Model file for the job. Use its own axes, mm. A direction names the side the tool comes from. Round coordinates to 2 decimals unless told otherwise and drop trailing zeros. Write each loop counter-clockwise with the first axis right and the second up, starting at its lowest first coordinate (ties: lowest second). Pieces come first, ordered by that corner, then holes.
```python
from build123d import *

# Parameters (mm, degrees)
SKETCH1_W                       = 210
SKETCH1_H                       = 120
CHASIS_BASE_DEPTH               = 3
FRONT_AND_BACK_SLOTS_DEPTH      = 279.202975413
FRONT_AND_BACK_SLOTS_DEPTH_BACK = 279.202975413
SKETCH7_W                       = 50
SKETCH7_H                       = 3
BACK_WHEELS_DEPTH               = 279.202975413
BACK_WHEELS_DEPTH_BACK          = 279.202975413
CUT_EXTRUDE1_DEPTH              = 279.202975413
CUT_EXTRUDE1_DEPTH_BACK         = 279.202975413
SKETCH16_W                      = 3
SKETCH16_H                      = 10.9
SKETCH17_W                      = 210
SKETCH17_H                      = 30.004914443
CUT_EXTRUDE2_DEPTH              = 10
SKETCH18_W                      = 80
SKETCH18_H                      = 65
CUT_EXTRUDE3_DEPTH              = 57
CUT_EXTRUDE4_DEPTH              = 10
BOSS_EXTRUDE1_DEPTH             = 3


with BuildPart() as part:
    # Sketch1 → Chasis Base (new body)
    with BuildSketch(Plane(origin=(0, 0, 0), x_dir=(1, 0, 0), z_dir=(0, 1, 0))):
        with Locations((-50.389260457, -170.742439233)):
            Rectangle(SKETCH1_W, SKETCH1_H)
    extrude(amount=CHASIS_BASE_DEPTH)

    # Sketch7 → Front and Back Slots (cut, two sides: drawn at the far end of the back side and taken through both)
    with BuildSketch(Plane(origin=(0, 3, 0), x_dir=(1, 0, 0), z_dir=(0, 1, 0)).offset(-FRONT_AND_BACK_SLOTS_DEPTH_BACK)):
        with Locations((-0.389260457, -229.242439233)):
            Rectangle(SKETCH7_W, SKETCH7_H)
        with Locations((-100.389260457, -229.242439233)):
            Rectangle(SKETCH7_W, SKETCH7_H)
    extrude(amount=FRONT_AND_BACK_SLOTS_DEPTH + FRONT_AND_BACK_SLOTS_DEPTH_BACK, mode=Mode.SUBTRACT)

    # Sketch15 → Back Wheels (cut, two sides: drawn at the far end of the back side and taken through both)
    with BuildSketch(Plane(origin=(0, 3, 0), x_dir=(1, 0, 0), z_dir=(0, 1, 0)).offset(-BACK_WHEELS_DEPTH_BACK)):
        Polygon((-155.389260457, -175.747353676), (-155.389260457, -140.747353676), (-127.889260457, -140.747353676), (-127.889260457, -210.747353676), (-155.389260457, -210.747353676), align=None)
        Polygon((54.610739543, -140.747353676), (27.110739543, -140.747353676), (27.110739543, -210.747353676), (54.610739543, -210.747353676), (54.610739543, -175.747353676), align=None)
    extrude(amount=BACK_WHEELS_DEPTH + BACK_WHEELS_DEPTH_BACK, mode=Mode.SUBTRACT)

    # Sketch16 → Cut-Extrude1 (cut, two sides: drawn at the far end of the back side and taken through both)
    with BuildSketch(Plane(origin=(0, 3, 0), x_dir=(1, 0, 0), z_dir=(0, 1, 0)).offset(-CUT_EXTRUDE1_DEPTH_BACK)):
        with Locations((-104.589260457, -155.177353676)):
            Rectangle(SKETCH16_W, SKETCH16_H)
        with Locations((3.810739543, -155.177353676)):
            Rectangle(SKETCH16_W, SKETCH16_H)
    extrude(amount=CUT_EXTRUDE1_DEPTH + CUT_EXTRUDE1_DEPTH_BACK, mode=Mode.SUBTRACT)

    # Sketch17 → Cut-Extrude2 (cut)
    with BuildSketch(Plane(origin=(0, 3, 0), x_dir=(1, 0, 0), z_dir=(0, 1, 0))):
        with Locations((-50.389260457, -125.744896455)):
            Rectangle(SKETCH17_W, SKETCH17_H)
    extrude(amount=-CUT_EXTRUDE2_DEPTH, mode=Mode.SUBTRACT)

    # Sketch18 → Cut-Extrude3 (cut)
    with BuildSketch(Plane(origin=(0, 0, 0), x_dir=(-1, 0, 0), z_dir=(0, -1, 0))):
        with Locations((50.389260457, -173.247353676)):
            Rectangle(SKETCH18_W, SKETCH18_H)
    extrude(amount=-CUT_EXTRUDE3_DEPTH, mode=Mode.SUBTRACT)

    # Sketch19 → Cut-Extrude4 (cut)
    with BuildSketch(Plane(origin=(0, 3, 0), x_dir=(1, 0, 0), z_dir=(0, 1, 0))):
        with BuildLine():
            Line((-155.389260457, -221.353955394), (-155.389260457, -210.747353676))
            Line((-155.389260457, -210.747353676), (-144.782658739, -210.747353676))
            ThreePointArc((-144.782658739, -210.747353676), (-152.282658739, -213.853955394), (-155.389260457, -221.353955394))
        make_face()
        with BuildLine():
            Line((-127.889260457, -140.747353676), (-117.282658739, -140.747353676))
            ThreePointArc((-117.282658739, -140.747353676), (-124.782658739, -143.853955394), (-127.889260457, -151.353955394))
            Line((-127.889260457, -151.353955394), (-127.889260457, -140.747353676))
        make_face()
        with BuildLine():
            Line((-90.389260457, -151.353955394), (-90.389260457, -140.747353676))
            Line((-90.389260457, -140.747353676), (-100.995862174, -140.747353676))
            ThreePointArc((-100.995862174, -140.747353676), (-93.495862174, -143.853955394), (-90.389260457, -151.353955394))
        make_face()
        with BuildLine():
            Line((-10.389260457, -140.747353676), (0.217341261, -140.747353676))
            ThreePointArc((0.217341261, -140.747353676), (-7.282658739, -143.853955394), (-10.389260457, -151.353955394))
            Line((-10.389260457, -151.353955394), (-10.389260457, -140.747353676))
        make_face()
        with BuildLine():
            Line((27.110739543, -151.353955394), (27.110739543, -140.747353676))
            Line((27.110739543, -140.747353676), (16.504137826, -140.747353676))
            ThreePointArc((16.504137826, -140.747353676), (24.004137826, -143.853955394), (27.110739543, -151.353955394))
        make_face()
        with BuildLine():
            Line((54.610739543, -210.747353676), (44.004137826, -210.747353676))
            ThreePointArc((44.004137826, -210.747353676), (51.504137826, -213.853955394), (54.610739543, -221.353955394))
            Line((54.610739543, -221.353955394), (54.610739543, -210.747353676))
        make_face()
    extrude(amount=-CUT_EXTRUDE4_DEPTH, mode=Mode.SUBTRACT)

    # Sketch20 → Boss-Extrude1 (add)
    with BuildSketch(Plane(origin=(0, 0, 0), x_dir=(1, 0, 0), z_dir=(0, 1, 0))):
        with BuildLine():
            Line((-90.389260457, -195.140751958), (-90.389260457, -205.747353676))
            Line((-90.389260457, -205.747353676), (-79.782658739, -205.747353676))
            ThreePointArc((-79.782658739, -205.747353676), (-87.282658739, -202.640751958), (-90.389260457, -195.140751958))
        make_face()
        with BuildLine():
            Line((-10.389260457, -205.747353676), (-20.995862174, -205.747353676))
            ThreePointArc((-20.995862174, -205.747353676), (-13.495862174, -202.640751958), (-10.389260457, -195.140751958))
            Line((-10.389260457, -195.140751958), (-10.389260457, -205.747353676))
        make_face()
    extrude(amount=BOSS_EXTRUDE1_DEPTH)


solid = part.part
```
1) Wall check: probe 1 along X at (y, z) = (1.4, 156.5); probe 2 along X at (y, z) = (0.3, 193); probe 3 along Z at (x, y) = (4.5, 2.8). Give the ranges that are in metal, low to high.
2) Flat gauge pins, fed straight in: pin 1 Ø1.5 at (y, z) = (2, 212) entering from -X; pin 2 Ø0.9 at (x, y) = (-43.5, 2) entering from -Z; pin 3 Ø0.9 at (x, y) = (-133, 2) entering from -Z; pin 4 Ø1 at (y, z) = (0.5, 221) entering from -X. Where does each tip first touch, or does it go through?
3) Cut at D-D on x = -137.5. List the corners of the cut face in (y, z), and give its area (3 significant figures).
4) Pull direction X, two halves, no side cores. Call faces 1 (the face through (51.42, 1.52, 213.77)), 2 (the face through (-124.7, 1.52, 143.77)), 3 (the face through (-93.58, 1.52, 143.77)): released by +X, released by -X, zero draft, split by the parting line, or undercut.
5) Cut at C-C on y = 2.5. Give the number of separate pieces and of enclosed holes in the cut face, and give its area (3 significant figures).
6) Which spindle directions (+Z, -Z, +X, -X, +Y, -Y) get a long thin tool onto all of the face, cutting with end or side? Do faces 4 (the face through (-7.2, 1.52, 143.77)), 5 (the face through (-52, 0, 215)). Say none if no direction does.
7) Cut at B-B on x = -65.5. List the corners of the cut face in (y, z).
8) Cut at A-A on z = 169.5. List the corners of the cut face in (x, y), and give its area (3 significant figures).
Result sheet:
1. probe 1: x = -127.89 to -106.09, -103.09 to -90.39, -10.39 to 2.31, 5.31 to 27.11
1. probe 2: x = -127.89 to -90.39, -10.39 to 27.11
1. probe 3: z = 140.75 to 149.73, 160.63 to 227.74
2. pin 1: stops at x = -150.99
2. pin 2: stops at z = 205.75
2. pin 3: stops at z = 210.75
2. pin 4: stops at x = -155.39
3. outline: (0, 210.75) - (3, 210.75) - (3, 230.74) - (0, 230.74) - close
3. area: 60.0 mm2
4. face 1: released by +X
4. face 2: released by -X
4. face 3: undercut
5. separate pieces: 1
5. enclosed holes: 2
5. area: 9,390 mm2
6. face 4: -Z, +Y, -Y
6. face 5: +Z, -Z, +X, -X, -Y
7. outline: (0, 205.75) - (3, 205.75) - (3, 230.74) - (0, 230.74) - close
8. outline: (-127.89, 0) - (-90.39, 0) - (-90.39, 3) - (-127.89, 3) - close; (-10.39, 0) - (27.11, 0) - (27.11, 3) - (-10.39, 3) - close
8. area: 225 mm2
